```python
from build123d import *

# Parameters (mm, degrees)
SKETCH1_R               = 3.55
BOSS_EXTRUDE1_DEPTH     = 5
CUT_EXTRUDE1_DEPTH      = 1.2
SKETCH3_R               = 8.75
BOSS_EXTRUDE2_DEPTH     = 3.5
CUT_EXTRUDE2_DEPTH      = 51.012898336
CUT_EXTRUDE2_DEPTH_BACK = 51.012898336
SKETCH5_R               = 0.6


with BuildPart() as part:
    # Sketch1 → Boss-Extrude1 (new body)
    with BuildSketch(Plane.XY):
        with BuildLine():
            Line((2.939387691, -45.6), (11.757550765, -2.4))
            ThreePointArc((11.757550765, -2.4), (-0.411368636, 11.992946921), (-11.565465836, -3.2))
            Line((-11.565465836, -3.2), (-0.8, -42.108633541))
            ThreePointArc((-0.8, -42.108633541), (-2.047353135, -47.192793912), (2.939387691, -45.6))
        make_face()
        Circle(SKETCH1_R, mode=Mode.SUBTRACT)
        with BuildLine():
            Line((1.321479166, -38.526100673), (7.223456236, -9.612436083))
            ThreePointArc((7.223456236, -9.612436083), (0.272467701, -12.215673533), (-6.678520834, -9.612436083))
            Line((-6.678520834, -9.612436083), (1.321479166, -38.526100673))
        make_face(mode=Mode.SUBTRACT)
    extrude(amount=BOSS_EXTRUDE1_DEPTH)

    # Sketch2 → Cut-Extrude1 (cut)
    with BuildSketch(Plane(origin=(0, 0, 0), x_dir=(-1, 0, 0), z_dir=(0, 0, -1))):
        with BuildLine():
            Line((-1.9821425, -15.266666667), (-3.964284999, -0.533333333))
            ThreePointArc((-3.964284999, -0.533333333), (0, 4), (3.964284999, -0.533333333))
            Line((3.964284999, -0.533333333), (1.9821425, -15.266666667))
            ThreePointArc((1.9821425, -15.266666667), (0, -17), (-1.9821425, -15.266666667))
        make_face()
    extrude(amount=-CUT_EXTRUDE1_DEPTH, mode=Mode.SUBTRACT)

    # Sketch3 → Boss-Extrude2 (add)
    with BuildSketch(Plane.XY.offset(5)):
        with BuildLine():
            ThreePointArc((11.757550765, -2.4), (-0.411368636, 11.992946921), (-11.565465836, -3.2))
            ThreePointArc((-11.565465836, -3.2), (0.411368636, -11.992946921), (11.757550765, -2.4))
        make_face()
        Circle(SKETCH3_R, mode=Mode.SUBTRACT)
    extrude(amount=BOSS_EXTRUDE2_DEPTH)

    # Sketch5 → Cut-Extrude2 (cut, two sides: drawn at the far end of the back side and taken through both)
    with BuildSketch(Plane(origin=(0, 0, 1.2), x_dir=(-1, 0, 0), z_dir=(0, 0, -1)).offset(-CUT_EXTRUDE2_DEPTH_BACK)):
        with Locations((-0.141802358, -6.414025874)):
            Circle(SKETCH5_R)
        with Locations((-0.086177178, -8.414025874)):
            Circle(SKETCH5_R)
        with Locations((0.232439079, -14.448130401)):
            Circle(SKETCH5_R)
        with Locations((0.20026758, -12.448389169)):
            Circle(SKETCH5_R)
    extrude(amount=CUT_EXTRUDE2_DEPTH + CUT_EXTRUDE2_DEPTH_BACK, mode=Mode.SUBTRACT)


solid = part.part
```
The listing builds one solid part. Answer for the finished solid, in the listing's coordinates (mm). A direction names the side the tool comes from. Give positions to 0.01 mm unless a question says otherwise; leave off trailing zeros. Order: outer loops, then holes, each group sorted by start corner. A loop starts at its lowest first (then second) coordinate and runs counter-clockwise, first axis right, second up. Notation, with made-up numbers: (27.5, 40.5) -> (47.5, 40.5) arc R18 cw to (47.5, 74.5) -> close; hole circle Ø2 at (17, 64). An arc over 180 degrees is marked (long way). One line per item, written item: value.
1) A tool of negligible diameter and unlimited length cuts with its end or side. For faces 1 (the flat face through (-6.26, -22.38, 2.46)), 2 (the flat face through (3.182, -6.344, 0.592)), 3 (the cylindrical face through (-0.18, -11.85, 4.09)), 4 (the flat face through (-3, -11, 0)), from which of +Z, -Z, +X, -X, +Y, -Y can it reach the whole face along a straight path? Write none if from no direction.
Reported:
face 1: +Z, -Z, -X
face 2: -Z
face 3: +Z, -Z
face 4: -Z, +X, -X, +Y, -Y
2) Find section D-D, the plane y = -45. Determine the outline of the cut face in (x, z).
Reported:
outline: (-3, 0) -> (3.06, 0) -> (3.06, 5) -> (-3, 5) -> close
3) Find section B-B, the plane x = 6. Determine the outline of the cut face in (y, z).
Reported:
outline: (-30.61, 0) -> (-15.61, 0) -> (-15.61, 5) -> (-30.61, 5) -> close; (-10.53, 0) -> (10.39, 0) -> (10.39, 8.5) -> (6.37, 8.5) -> (6.37, 5) -> (-6.37, 5) -> (-6.37, 8.5) -> (-10.39, 8.5) -> (-10.39, 5) -> (-10.53, 5) -> close
4) Find section C-C, the plane z = 3.25. Determine the outline of the cut face in (x, y).
Reported:
outline: (-11.57, -3.2) -> (-0.8, -42.11) arc R3 ccw (long way) to (2.94, -45.6) -> (11.76, -2.4) arc R12 ccw (long way) to start; hole (-6.68, -9.61) -> (1.32, -38.53) -> (7.22, -9.61) arc R10.58 cw to (0.35, -12.22) arc R0.6 ccw to (-0.73, -12.17) arc R10.58 cw to start; hole circle Ø7.1 at (0, 0); hole circle Ø1.2 at (0.09, -8.41); hole circle Ø1.2 at (0.14, -6.41)
5) Find section A-A, the plane y = -32. Determine the outline of the cut face in (x, z).
Reported:
outline: (-3.6, 0) -> (-0.48, 0) -> (-0.48, 5) -> (-3.6, 5) -> close; (2.65, 0) -> (5.72, 0) -> (5.72, 5) -> (2.65, 5) -> close
6) Find the intervals of material crossed by line 1 (X direction, y = -11, z = 1.5); line 2 (Z direction, x = -6.75, y = -19); line 3 (X direction, y = 0, z = 5.7), in increasing order.
Reported:
line 1: x = -9.41 to -6.29, -4.65 to 5.2, 6.94 to 10
line 2: z = 0 to 5
line 3: x = -12 to -8.75, 8.75 to 12
7) Flat-ended cylindrical pins translate along their axes: P1, Ø5, axis at x = -3.5, z = 4, coming from the -Y side; P2, Ø1, axis at x = -5, z = 6, coming from the +Y side; P3, Ø8, axis at x = 0, y = 0, coming from the +Z side. Find the tip coordinate at first contact, or state that the pin passes through.
Reported:
P1: stops at y = -47.83
P2: stops at y = 11.12
P3: stops at z = 5
8) Determine the mould class of faces 5 (the cylindrical face through (-3.863, -11.374, 2.465)), 6 (the flat face through (7.287, -24.302, 2.465)), 7 (the flat face through (-1, -9, 8.5)), 8 (the flat face through (0, -4, 5)) for opening direction Y: pulls with the +Y half, pulls with the -Y half, needs draft (parallel to the pull), parting line crosses it, or undercut.
Reported:
face 5: undercut
face 6: pulls with the -Y half
face 7: needs draft
face 8: undercut
